Input: part model. Units: mm. Frame: model coordinates. A direction names the side the tool comes from. Coordinates: 2 decimals unless noted, no trailing zeros.
(1) Section A-A, the plane y = 3. Give the number of separate pieces and of enclosed holes in the cut face, then the cut area to 3 significant figures.
(2) Line query: L1, parallel to X at y = 2, z = 2.2; L2, parallel to X at y = -40, z = 0.45; L3, parallel to Y at x = 36.5, z = 1.45. Output: solid intervals per line, ascending.
(3) Set-up query: faces 4 (the face through (27.49, 1.56, 1.48)), 5 (the face through (36.083, -8.469, 1.482)), 6 (the face through (71.501, -24.226, 2.877)), 7 (the face through (54.363, -10.398, 1.521)), 8 (the face through (71.35, -24.16, 1.48)). Return all of +Z, -Z, +X, -X, +Y, -Y with unobstructed straight access to the full face (end or side cutting, diameter ignored); none if empty.
(4) Mould query, pull axis Y, two halves, no side actions, for faces 1 (the face through (73.8, -21.81, 1.48)), 2 (the face through (10.492, 1.597, 2.877)), 3 (the face through (48.747, -11.064, 1.521)). Classes: released by +Y, released by -Y, zero draft, split by the parting line, or undercut.
(5) Contact query for a flat-ended pin moving along its axis: P1, Ø2.5, axis at x = 13, y = 3, coming from the -Z side. Output: stop coordinate, or through.
```python
from build123d import *
from OCP.BRepFilletAPI import BRepFilletAPI_MakeFillet

# Parameters (mm, degrees)
EXTRUDE_THIN1_DEPTH     = 3
SKETCH1_6_R             = 3
BOSS_EXTRUDE2_DEPTH     = 3
FILLET1_R               = 10
FILLET2_R               = 10
FILLET3_R1              = 10
FILLET3_R2              = 5
CHAMFER1_SIZE           = 0.25
CUT_EXTRUDE1_DEPTH      = 90.36389433
F_3_0_MM_DOWEL_HOLES1_D = 3


with BuildPart() as part:
    # Sketch1 → Extrude-Thin1 (new body)
    with BuildSketch(Plane.XY):
        with BuildLine():
            ThreePointArc((13.956778483, 1.844761957), (18.364214045, 3.961300509), (23.249537827, 3.764233943))
            ThreePointArc((23.249537827, 3.764233943), (27.544341573, 1.513827454), (30.636293504, -2.221075738))
            ThreePointArc((30.636293504, -2.221075738), (36.280115015, -8.611383188), (44.176022564, -11.827498007))
            Line((44.176022564, -11.827498007), (64.112853909, -14.973721748))
            ThreePointArc((64.112853909, -14.973721748), (67.995089498, -16.803438115), (70.284091708, -20.433876661))
            Line((70.284091708, -20.433876661), (73.760858733, -32.587064718))
            Line((73.760858733, -32.587064718), (76.645152845, -31.761929896))
            Line((76.645152845, -31.761929896), (73.168385821, -19.60874184))
            ThreePointArc((73.168385821, -19.60874184), (69.983011914, -14.556626047), (64.580495529, -12.010394005))
            Line((64.580495529, -12.010394005), (44.643664184, -8.864170263))
            ThreePointArc((44.643664184, -8.864170263), (38.016065461, -6.164655567), (33.278803277, -0.80081446))
            ThreePointArc((33.278803277, -0.80081446), (29.432995007, 3.844704587), (24.091064686, 6.64378817))
            ThreePointArc((24.091064686, 6.64378817), (17.757357703, 6.899280322), (12.043221517, 4.155238043))
            Line((12.043221517, 4.155238043), (13.956778483, 1.844761957))
        make_face()
    extrude(amount=EXTRUDE_THIN1_DEPTH)

    # Sketch1<6> → Boss-Extrude2 (add)
    with BuildSketch(Plane.XY):
        with BuildLine():
            ThreePointArc((78.472958706, -32.673622319), (75.046124973, -34.175890794), (72.819900547, -31.168578904))
            ThreePointArc((72.819900547, -31.168578904), (72.324756821, -34.48620054), (71.104744395, -37.610836569))
            ThreePointArc((71.104744395, -37.610836569), (74.47911855, -36.0951074), (76.759757859, -39.007584043))
            ThreePointArc((76.759757859, -39.007584043), (76.759268993, -39.061740839), (76.757802553, -39.115879984))
            ThreePointArc((76.757802553, -39.115879984), (77.252946279, -35.798258348), (78.472958706, -32.673622319))
        make_face()
        with BuildLine():
            ThreePointArc((78.817945242, -31.276874845), (77.878853444, -29.096815814), (75.649506987, -28.281607152))
            Line((75.649506987, -28.281607152), (76.645152845, -31.761929896))
            Line((76.645152845, -31.761929896), (75.203005789, -32.174497307))
            Line((75.203005789, -32.174497307), (73.760858733, -32.587064718))
            Line((73.760858733, -32.587064718), (73.053014062, -30.112763351))
            ThreePointArc((73.053014062, -30.112763351), (72.888498306, -30.63008226), (72.819900547, -31.168578904))
            ThreePointArc((72.819900547, -31.168578904), (75.046124973, -34.175890794), (78.472958706, -32.673622319))
            ThreePointArc((78.472958706, -32.673622319), (78.730421885, -31.996235537), (78.817945242, -31.276874845))
        make_face()
        with Locations((73.759757859, -39.007584043)):
            Circle(SKETCH1_6_R)
        with Locations((13, 3)):
            Circle(SKETCH1_6_R)
        Polygon((46.29255307, -8.112005426), (62.855890569, -10.725859392), (62.07648787, -15.664738964), (45.51315037, -13.050884998), align=None)
    extrude(amount=BOSS_EXTRUDE2_DEPTH)

    # Fillet1
    # the kernel refuses this fillet: 10 mm, written as the material it takes off along each edge
    with BuildSketch(Plane(origin=(45.51315037, -13.050884998, -10.897247359), x_dir=(0.9877759145103069, -0.1558805398801499, 0), z_dir=(0, 0, 1)), Plane(origin=(62.855890569, -10.725859392, -10.897247359), x_dir=(-0.9877759145103069, 0.15588053988014952, 0), z_dir=(0, 0, 1))) as fillet1_piece_1:
        with BuildLine():
            CenterArc((4.358898944, 10), FILLET1_R, 244.158067237, 25.841932763)
            Line((0, 1), (-0.087177979, 0.82))
            ThreePointArc((-0.087177979, 0.82), (-0.2, 0.5), (-0.2, 0))
            Line((-0.2, 0), (0, -0.2))
            Line((0, -0.2), (4.358898944, -0.2))
            Line((4.358898944, -0.2), (4.358898944, 0))
        make_face()
    extrude(amount=24.794494718, mode=Mode.SUBTRACT)
    with BuildSketch(Plane(origin=(62.07648787, -15.664738964, -10.897247359), x_dir=(0.1558805398801516, 0.9877759145103067, 0), z_dir=(0, 0, 1)), Plane(origin=(46.29255307, -8.112005426, -10.897247359), x_dir=(-0.1558805398801516, -0.9877759145103067, 0), z_dir=(0, 0, 1))) as fillet1_piece_2:
        with BuildLine():
            CenterArc((10, 4.358898944), FILLET1_R, 180, 25.841932763)
            Line((0, 4.358898944), (-0.2, 4.358898944))
            Line((-0.2, 4.358898944), (-0.2, 0))
            Line((-0.2, 0), (0, -0.2))
            ThreePointArc((0, -0.2), (0.5, -0.2), (0.82, -0.087177979))
            Line((0.82, -0.087177979), (1, 0))
        make_face()
    extrude(amount=24.794494718, mode=Mode.SUBTRACT)

    # Fillet2
    fillet2_edges = [part.edges().sort_by_distance(p)[0] for p in [
        (62.23236841, -14.67696305, 1.5),
        (62.70001003, -11.713635306, 1.5),
        (45.66903091, -12.063109084, 1.5),
        (46.13667253, -9.09978134, 1.5),
    ]]
    fillet(fillet2_edges, radius=FILLET2_R)

    # Fillet3: one fillet with a radius per group of edges: ONE call of the kernel's fillet builder (fillet() takes one radius for all edges)
    fillet3_edges_1 = [part.edges().sort_by_distance(p)[0] for p in [
        (73.053014062, -30.112763351, 1.5),
        (75.649506987, -28.281607152, 1.5),
    ]]
    fillet3_edges_2 = [part.edges().sort_by_distance(p)[0] for p in [
        (14.342872483, 5.682665371, 1.5),
        (15.99591873, 3.156431979, 1.5),
    ]]
    fillet3 = BRepFilletAPI_MakeFillet(part.part.solid().wrapped)
    for e in fillet3_edges_1:
        fillet3.Add(FILLET3_R1, e.wrapped)
    for e in fillet3_edges_2:
        fillet3.Add(FILLET3_R2, e.wrapped)
    add(Compound.cast(fillet3.Shape()), mode=Mode.REPLACE)

    # Chamfer1
    chamfer1_edges = [part.edges().sort_by_distance(p)[0] for p in [
        (54.57422182, -9.418932409, 0),
        (60.092477637, -10.417114134, 0),
        (48.27462413, -13.358997517, 0),
        (54.57422182, -9.418932409, 3),
        (49.025073316, -8.669242301, 3),
        (59.352291729, -15.107486729, 3),
        (29.432995007, 3.844704587, 0),
        (48.27462413, -13.358997517, 3),
        (64.571774389, -12.009017725, 0),
        (36.178802299, -8.53899299, 0),
        (36.178802299, -8.53899299, 3),
        (37.633792223, -5.884652293, 0),
        (37.633792223, -5.884652293, 3),
        (21.456361373, 4.116360797, 3),
        (69.983011914, -14.556626047, 0),
        (49.025073316, -8.669242301, 0),
        (59.352291729, -15.107486729, 0),
        (60.092477637, -10.417114134, 3),
        (45.406180886, -12.157630236, 0),
        (45.406180886, -12.157630236, 3),
        (45.57735687, -8.918557885, 0),
        (45.57735687, -8.918557885, 3),
        (62.513992379, -14.848753903, 0),
        (67.995089498, -16.803438115, 0),
        (62.513992379, -14.848753903, 3),
        (63.02085079, -11.636919182, 0),
        (63.02085079, -11.636919182, 3),
        (64.104132769, -14.972345468, 0),
        (27.544341573, 1.513827454, 0),
        (21.456361373, 4.116360797, 0),
        (10.338658069, 1.615348734, 3),
        (19.856644471, 7.158769061, 0),
        (10.338658069, 1.615348734, 0),
        (73.788452871, -21.776212775, 0),
        (73.788452871, -21.776212775, 3),
        (71.36386404, -24.208267097, 0),
        (71.36386404, -24.208267097, 3),
        (72.820223354, -31.159983943, 0),
        (72.820223354, -31.159983943, 3),
        (17.30302071, 3.35546819, 0),
        (27.544341573, 1.513827454, 3),
        (17.30302071, 3.35546819, 3),
        (14.523458256, 5.993511964, 0),
        (14.523458256, 5.993511964, 3),
        (75.675797588, -26.700228887, 3),
        (75.675797588, -26.700228887, 0),
        (72.759314108, -29.551891496, 3),
        (72.759314108, -29.551891496, 0),
        (64.104132769, -14.972345468, 3),
        (67.995089498, -16.803438115, 3),
        (78.757105023, -30.675759401, 0),
        (77.252946279, -35.798258348, 0),
        (72.324756821, -34.48620054, 0),
        (72.987937591, -41.906599992, 0),
        (72.324756821, -34.48620054, 3),
        (72.987937591, -41.906599992, 3),
        (77.252946279, -35.798258348, 3),
        (78.757105023, -30.675759401, 3),
        (69.983011914, -14.556626047, 3),
        (64.571774389, -12.009017725, 3),
        (19.856644471, 7.158769061, 3),
        (29.432995007, 3.844704587, 3),
        (53.79481912, -14.357811981, 0),
        (53.79481912, -14.357811981, 3),
    ]]
    chamfer(chamfer1_edges, length=CHAMFER1_SIZE)

    # Sketch2 → Cut-Extrude1 (cut, through all)
    with BuildSketch(Plane.XY.offset(3)):
        with BuildLine():
            Line((50.467237622, -9.783186164), (58.369444938, -11.030230483))
            ThreePointArc((58.369444938, -11.030230483), (59.617288, -12.745715164), (57.901803318, -13.993558226))
            Line((57.901803318, -13.993558226), (49.999596002, -12.746513907))
            ThreePointArc((49.999596002, -12.746513907), (48.75175294, -11.031029225), (50.467237622, -9.783186164))
        make_face()
    extrude(amount=-CUT_EXTRUDE1_DEPTH, mode=Mode.SUBTRACT)

    # Ø3.0 mm Dowel Holes1 (through all)
    with Locations(Plane.XY.offset(3)):
        with Locations((13, 3), (75.817945242, -31.276874845), (73.759757859, -39.007584043)):
            Hole(F_3_0_MM_DOWEL_HOLES1_D / 2)


solid = part.part
```
Report:
1. separate pieces: 3
1. enclosed holes: 0
1. area: 26.6 mm2
2. L1: x = 10.17 to 11.88, 14.12 to 15.9, 26.9 to 31.34
2. L2: x = 70.93 to 72.63, 74.88 to 76.59
2. L3: y = -8.77 to -4.94
3. face 4: +Z, -Z, -Y
3. face 5: +Z, -Z, -X, -Y
3. face 6: +Z, -X
3. face 7: +Z, -Z
3. face 8: +Z, -Z, -X
4. face 1: released by +Y
4. face 2: split by the parting line
4. face 3: undercut
5. P1: passes through
